Check sheet for the modelled part. Datum: model origin and axes. Units: mm. Coordinates: 2 decimals unless noted, no trailing zeros. Write each loop counter-clockwise with the first axis right and the second up, starting at its lowest first coordinate (ties: lowest second). Pieces come first, ordered by that corner, then holes. Notation, with made-up numbers: (66.5, 2.25) - (111.5, 2.25) arc R13 ccw to (111.5, 24.25) - close; hole circle Ø3 at (12, 24.25). An arc over 180 degrees is marked (long way). Use one line per item in the form item = value. Start each with the question number.
1. Go/stop test with flat-tipped pins: pin 1 Ø6 at (x, z) = (3, -68) entering from +Y; pin 2 Ø6 at (x, z) = (2.5, -23) entering from -Y; pin 3 Ø3.5 at (y, z) = (0, 3) entering from +X. Record where each tip stops, or that it passes through.
2. Scan lines: line 1 along Z through (x, y) = (1.5, 3.5); line 2 along Y through (x, z) = (2.5, -98.5); line 3 along Y through (x, z) = (0.25, -105.5). Record each from-to range of solid material in increasing order.
3. Cross-section at C-C on z = -15. Record the boundary of the cut face in (x, y), then the cut area to 3 significant figures.
4. Cross-section at A-A on x = 0. Record the boundary of the cut face in (y, z), then the cut area to 3 significant figures.
5. Cross-section at B-B on y = 0. Record the boundary of the cut face in (x, z), then the cut area to 3 significant figures.
```python
from build123d import *

# Parameters (mm, degrees)
CUT_EXTRUDE1_DEPTH = 4


with BuildPart() as part:
    # Sketch1 → Revolve1 (revolve)
    with BuildSketch(Plane(origin=(0, 0, 0), x_dir=(0, 0, -1), z_dir=(1, 0, 0)), mode=Mode.PRIVATE) as revolve1_sk:
        Polygon((-5, 0), (-5, 3), (117.3, 3), (117.3, 6), (120.3, 6), (120.3, 0), align=None)
    revolve(revolve1_sk.sketch.rotate(Axis((0, 0, -120.3), (0, 0, 1)), 270), axis=Axis((0, 0, -120.3), (0, 0, 1)))

    # Sketch2 → Revolve2 (revolve)
    with BuildSketch(Plane(origin=(0, 0, 0), x_dir=(0, 0, -1), z_dir=(1, 0, 0)), mode=Mode.PRIVATE) as revolve2_sk:
        with BuildLine():
            Line((-21, 0), (-21, 2.3865))
            Line((-21, 2.3865), (-20.3865, 3))
            Line((-20.3865, 3), (-8.148486452, 3))
            Line((-8.148486452, 3), (-6.599415898, 2.436184428))
            ThreePointArc((-6.599415898, 2.436184428), (-6.498392718, 2.409115348), (-6.394203812, 2.4))
            Line((-6.394203812, 2.4), (-5.6, 2.4))
            ThreePointArc((-5.6, 2.4), (-5.175735931, 2.575735931), (-5, 3))
            Line((-5, 3), (-4, 3))
            Line((-4, 3), (-4, 0))
            Line((-4, 0), (-21, 0))
        make_face()
    revolve(revolve2_sk.sketch.rotate(Axis((0, 0, 4), (0, 0, 1)), 270), axis=Axis((0, 0, 4), (0, 0, 1)))

    # Sketch3 → Cut-Extrude1 (cut)
    with BuildSketch(Plane.XY.offset(2)):
        Polygon((-5, 10), (-5, -5), (-2.5, -5), (-2.5, 5), (2.5, 5), (2.5, -5), (5, -5), (5, 10), align=None)
    extrude(amount=CUT_EXTRUDE1_DEPTH, mode=Mode.SUBTRACT)


solid = part.part
```
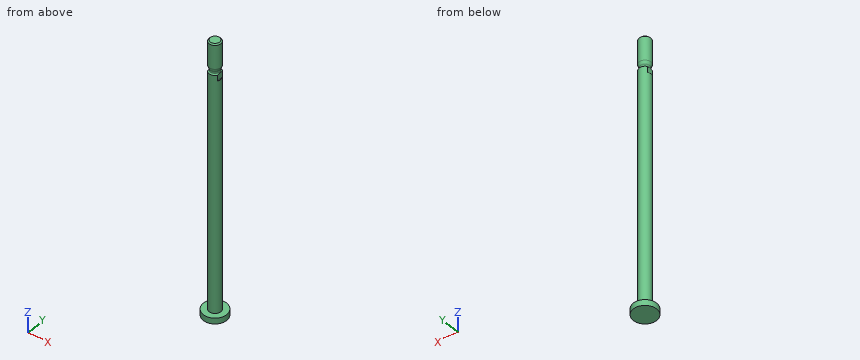
Final values:
q1.pin_1 = 3
q1.pin_2 = -3
q1.pin_3 = 3
q2.line_1 = -120.3 to -117.3
q2.line_2 = -1.66 to 1.66
q2.line_3 = -2.99 to 2.99
q3.outline = circle Ø6 at (0, 0)
q3.area = 28.3 mm²
q4.outline = (-6, -120.3) - (6, -120.3) - (6, -117.3) - (3, -117.3) - (3, 5) arc R0.6 cw to (2.4, 5.6) - (2.4, 6.39) arc R0.6 cw to (2.44, 6.6) - (3, 8.15) - (3, 20.39) - (2.39, 21) - (-2.39, 21) - (-3, 20.39) - (-3, 8.15) - (-2.44, 6.6) arc R0.6 cw to (-2.4, 6.39) - (-2.4, 5.6) arc R0.6 cw to (-3, 5) - (-3, -117.3) - (-6, -117.3) - close
q4.area = 863 mm²
q5.outline = (-6, -120.3) - (6, -120.3) - (6, -117.3) - (3, -117.3) - (3, 2) - (2.5, 2) - (2.5, 5.27) arc R0.6 cw to (2.4, 5.6) - (2.4, 6.39) arc R0.6 cw to (2.44, 6.6) - (3, 8.15) - (3, 20.39) - (2.39, 21) - (-2.39, 21) - (-3, 20.39) - (-3, 8.15) - (-2.44, 6.6) arc R0.6 cw to (-2.4, 6.39) - (-2.4, 5.6) arc R0.6 cw to (-2.5, 5.27) - (-2.5, 2) - (-3, 2) - (-3, -117.3) - (-6, -117.3) - close
q5.area = 860 mm²
